from build123d import *

# Parameters (mm, degrees)
SKETCH_1_W      = 180
SKETCH_1_H      = 180
SKETCH_1_R      = 1.9
SKETCH_1_R_2    = 30
EXTRUDE_1_DEPTH = 4
FILLET_1_R      = 20


with BuildPart() as part:
    # Эскиз1 → Бобышка-Вытянуть1 (new body)
    with BuildSketch(Plane(origin=(0, 0, 0), x_dir=(1, 0, 0), z_dir=(0, 1, 0))):
        Rectangle(SKETCH_1_W, SKETCH_1_H)
        with Locations(Location((-75, 82, 0), (0, 0, 270))):
            Circle(SKETCH_1_R, mode=Mode.SUBTRACT)
        with Locations(Location((-82, 75, 0), (0, 0, 270))):
            Circle(SKETCH_1_R, mode=Mode.SUBTRACT)
        with Locations(Location((82, 75, 0), (0, 0, 90))):
            Circle(SKETCH_1_R, mode=Mode.SUBTRACT)
        with Locations(Location((75, 82, 0), (0, 0, 90))):
            Circle(SKETCH_1_R, mode=Mode.SUBTRACT)
        with Locations(Location((75, -82, 0), (0, 0, 270))):
            Circle(SKETCH_1_R, mode=Mode.SUBTRACT)
        with Locations(Location((82, -75, 0), (0, 0, 270))):
            Circle(SKETCH_1_R, mode=Mode.SUBTRACT)
        with Locations(Location((-82, -75, 0), (0, 0, 90))):
            Circle(SKETCH_1_R, mode=Mode.SUBTRACT)
        with Locations(Location((-75, -82, 0), (0, 0, 90))):
            Circle(SKETCH_1_R, mode=Mode.SUBTRACT)
        with Locations(Location((20.859650045, 20.859650045, 0), (0, 0, 270))):
            Circle(SKETCH_1_R, mode=Mode.SUBTRACT)
        with Locations(Location((20.859650045, -20.859650045, 0), (0, 0, 270))):
            Circle(SKETCH_1_R, mode=Mode.SUBTRACT)
        with Locations(Location((-20.859650045, -20.859650045, 0), (0, 0, 270))):
            Circle(SKETCH_1_R, mode=Mode.SUBTRACT)
        with Locations(Location((-20.859650045, 20.859650045, 0), (0, 0, 270))):
            Circle(SKETCH_1_R, mode=Mode.SUBTRACT)
        with Locations(Location((-50, 50, 0), (0, 0, 270))):
            Circle(SKETCH_1_R_2, mode=Mode.SUBTRACT)
        with Locations(Location((50, 50, 0), (0, 0, 90))):
            Circle(SKETCH_1_R_2, mode=Mode.SUBTRACT)
        with Locations(Location((-50, -50, 0), (0, 0, 90))):
            Circle(SKETCH_1_R_2, mode=Mode.SUBTRACT)
        with Locations(Location((50, -50, 0), (0, 0, 270))):
            Circle(SKETCH_1_R_2, mode=Mode.SUBTRACT)
    extrude(amount=EXTRUDE_1_DEPTH)

    # Скругление1
    fillet_1_edges = [part.edges().sort_by_distance(p)[0] for p in [
        (90, 2, 90),
        (-90, 2, 90),
        (-90, 2, -90),
        (90, 2, -90),
    ]]
    fillet(fillet_1_edges, radius=FILLET_1_R)


solid = part.part
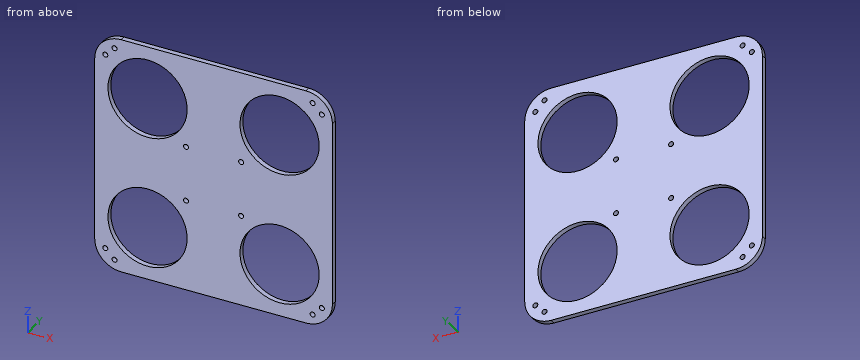
Model file for the job. Use its own axes, mm. Give positions to 0.01 mm unless a question says otherwise; leave off trailing zeros. Write each loop counter-clockwise with the first axis right and the second up, starting at its lowest first coordinate (ties: lowest second). Pieces come first, ordered by that corner, then holes. Notation, with made-up numbers: (50.5, 49) -> (70.5, 49) arc R7 cw to (70.5, 61) -> close; hole circle Ø7 at (50.25, -18). An arc over 180 degrees is marked (long way). Write item = value, one per line.
(1) Slice it at B-B, the plane x = 50. Give the cut face in (y, z), then the cut area to 3 significant figures.
Determined:
outline = (0, -90) -> (4, -90) -> (4, -80) -> (0, -80) -> close; (0, -20) -> (4, -20) -> (4, 20) -> (0, 20) -> close; (0, 80) -> (4, 80) -> (4, 90) -> (0, 90) -> close
area = 240 mm2
(2) Slice it at A-A, the plane z = -50. Give the cut face in (x, y), then the cut area to 3 significant figures.
Determined:
outline = (-90, 0) -> (-80, 0) -> (-80, 4) -> (-90, 4) -> close; (-20, 0) -> (20, 0) -> (20, 4) -> (-20, 4) -> close; (80, 0) -> (90, 0) -> (90, 4) -> (80, 4) -> close
area = 240 mm2
(3) Probe line 1 along X through (y, z) = (1.85, 50); line 2 along Z through (x, y) = (76, 0.45); line 3 along Z through (x, y) = (58.5, 1.85). List the from-to ranges inside material, lowest first.
Determined:
line_1 = -90 to -80, -20 to 20, 80 to 90
line_2 = -89.08 to -83.62, -80.38 to -64.97, -35.03 to 35.03, 64.97 to 80.38, 83.62 to 89.08
line_3 = -90 to -78.77, -21.23 to 21.23, 78.77 to 90
(4) Slice it at C-C, the plane y = 3.4. Give the number of separate pieces and of enclosed holes in the cut face, then the cut area to 3 significant figures.
Determined:
separate_pieces = 1
enclosed_holes = 16
area = 20,600 mm2
(5) Flat gauge pin, fed straight in: P1, Ø2.5, axis at x = -20.86, z = 20.86, coming from the +Y side. Where does the tip first touch, or does it go through?
Determined:
P1 = through
